The model under review builds one solid part; all positions refer to its coordinate system, in mm. Face numbers are marked on the shaded views. A direction names the side the tool comes from. Give positions to 0.01 mm unless a question says otherwise; leave off trailing zeros. Loops run counter-clockwise (first coordinate to the right, second up) from the corner with the lowest first, then second, coordinate; pieces in that order, holes last. Notation, with made-up numbers: (6, -25) - (13, -25) arc R23 ccw to (13, 0) - close; hole circle Ø2 at (-19, 40). An arc over 180 degrees is marked (long way). Answer as a JSON object with one key per item and string values.
from build123d import *

# Parameters (mm, degrees)
F0_W      = 31.8516
F0_H      = 7.8232
F1_DEPTH  = 9.6012
F2_R      = 2.4511
F3_DEPTH  = 1.905
F4_R      = 2.4511
F5_DEPTH  = 1.905
F6_R      = 2.4511
F7_DEPTH  = 1.905
F8_W      = 28.702
F8_H      = 4.572
F9_DEPTH  = 7.62
F10_R     = 1.5113
F11_DEPTH = 7.62


with BuildPart() as f1:
    # F0 (on Top) → F1 (new body)
    with BuildSketch(Plane.XY):
        Rectangle(F0_W, F0_H)
    extrude(amount=F1_DEPTH)

    # F2 (on face) → F3 (join)
    with BuildSketch(Plane.XY.offset(9.6012)):
        with Locations((-11.6967, 0)):
            Circle(F2_R)
    extrude(amount=F3_DEPTH)

    # F4 (on face) → F5 (join)
    with BuildSketch(Plane.XY.offset(9.6012)):
        with Locations((11.6967, 0.0635)):
            Circle(F4_R)
    extrude(amount=F5_DEPTH)

    # F6 (on face) → F7 (join)
    with BuildSketch(Plane.XY.offset(9.6012)):
        with Locations((-3.721353, 0.0635)):
            Circle(F6_R)
        with Locations((3.7211, 0.0635)):
            Circle(F6_R)
    extrude(amount=F7_DEPTH)

    # F8 (on face) → F9 (cut)
    with BuildSketch(Plane(origin=(0, 0, 0), x_dir=(1, 0, 0), z_dir=(0, 0, -1))):
        Rectangle(F8_W, F8_H)
    extrude(amount=-F9_DEPTH, mode=Mode.SUBTRACT)

    # F10 (on face) → F11 (join)
    with BuildSketch(Plane(origin=(0, 0, 7.62), x_dir=(1, 0, 0), z_dir=(0, 0, -1))):
        Circle(F10_R)
        with Locations((-7.9248, 0)):
            Circle(F10_R)
        with Locations((7.9248, 0)):
            Circle(F10_R)
    extrude(amount=F11_DEPTH)


solid = f1.part
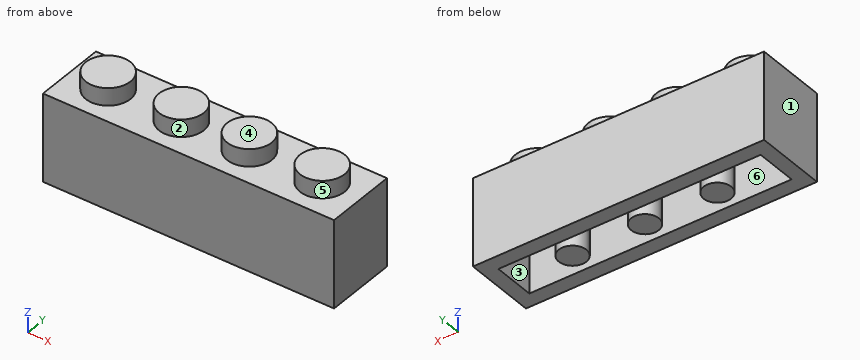
Q1. Consider section B-B, the plane x = 0. State the section outline as (y, z) points.
Results:
{"outline": "(-3.91, 0) - (-2.29, 0) - (-2.29, 7.62) - (-1.51, 7.62) - (-1.51, 0) - (1.51, 0) - (1.51, 7.62) - (2.29, 7.62) - (2.29, 0) - (3.91, 0) - (3.91, 9.6) - (-3.91, 9.6) - close"}
Q2. To check wall thickness, follow probe 1 along Y at (x, z) = (12.5, 4.5); probe 2 along X at (y, z) = (-2, 5); probe 3 along Y at (x, z) = (-8.5, 4.5). State the ranges of each line that lie inside material, in increasing order. Write a range as [from, to].
Results:
{"probe 1": "y = [-3.91, -2.29], [2.29, 3.91]", "probe 2": "x = [-15.93, -14.35], [14.35, 15.93]", "probe 3": "y = [-3.91, -2.29], [-1.4, 1.4], [2.29, 3.91]"}
Q3. Consider section C-C, the plane y = -3.25. State the section outline as (x, z) points.
Results:
{"outline": "(-15.93, 0) - (15.93, 0) - (15.93, 9.6) - (-15.93, 9.6) - close"}
Q4. Consider section A-A, the plane z = 1.75. State the section outline as (x, y) points.
Results:
{"outline": "(-15.93, -3.91) - (15.93, -3.91) - (15.93, 3.91) - (-15.93, 3.91) - close; circle Ø3.02 at (-7.92, 0); circle Ø3.02 at (0, 0); circle Ø3.02 at (7.92, 0); hole (-14.35, -2.29) - (14.35, -2.29) - (14.35, 2.29) - (-14.35, 2.29) - close"}
Q5. The part is to be moulded in two halves that separate along Y. For the marked faces 1, 2 and 3, say which applies: +Y half, -Y half, draft (parallel to the pull), parting line (faces both ways), or undercut.
Results:
{"face 1": "draft", "face 2": "parting line", "face 3": "undercut"}
Q6. Clearance check with a flat-ended pin moving along its axis: pin 1 Ø3 at (x, y) = (-7.5, 3) entering from +Z. State where the tip first meets the part, or that it passes through.
Results:
{"pin 1": "stops at z = 9.6"}
Q7. For the marked faces 4, 5 and 6, list the 3-axis set-ups (+Z, -Z, +X, -X, +Y, -Y) from which the entire face can be reached by the end or side of a thin tool; tool diameter is ignored.
Results:
{"face 4": "+Z, +X, -X, +Y, -Y", "face 5": "+Z", "face 6": "-Z"}
